Here's how the part is built. I have some questions about the finished solid (model axes, mm). A direction names the side the tool comes from. Round coordinates to 2 decimals unless told otherwise and drop trailing zeros. Order: outer loops, then holes, each group sorted by start corner. A loop starts at its lowest first (then second) coordinate and runs counter-clockwise, first axis right, second up. Notation, with made-up numbers: (34.5, -27) -> (66.5, -27) arc R9 cw to (66.5, -13) -> close; hole circle Ø5 at (-8, -22). An arc over 180 degrees is marked (long way). Answer in a Markdown table with one row per item.
```python
from build123d import *

# Parameters (mm, degrees)
SKETCH1_R           = 22.5
BOSS_EXTRUDE1_DEPTH = 8
CUT_EXTRUDE4_DEPTH  = 111.127199183


with BuildPart() as part:
    # Sketch1 → Boss-Extrude1 (new body)
    with BuildSketch(Plane(origin=(0, 0, 0), x_dir=(1, 0, 0), z_dir=(0, 1, 0))):
        Polygon((10, 0), (35, 0), (35, 8), (60, 8), (60, 92), (35, 92), (35, 100), (10, 100), (10, 92), (0, 92), (0, 8), (10, 8), align=None)
        with Locations(Location((30, 50, 0), (0, 0, 270))):
            Circle(SKETCH1_R, mode=Mode.SUBTRACT)
    extrude(amount=BOSS_EXTRUDE1_DEPTH)

    # Sketch7 → Cut-Extrude4 (cut, through all)
    with BuildSketch(Plane.XY.offset(-8)):
        Polygon((60, 0), (52, 8), (60, 8), align=None)
    extrude(amount=-CUT_EXTRUDE4_DEPTH, mode=Mode.SUBTRACT)


solid = part.part
```
1. Please list where these lines run through material, in increasing order: line 1 along Z through (x, y) = (30, 4.5); line 2 along Z through (x, y) = (28, 5); line 3 along X through (y, z) = (2.5, -50).
Numbers:
| item | result |
|---|---|
| line 1 | z = -100 to -72.5, -27.5 to 0 |
| line 2 | z = -100 to -72.41, -27.59 to 0 |
| line 3 | x = 0 to 7.5, 52.5 to 57.5 |
2. For pin 1 Ø4 at (y, z) = (5.5, -4) entering from -X; pin 2 Ø4 at (x, y) = (5, 6) entering from -Z; pin 3 Ø1.5 at (x, y) = (53, 5) entering from +Z, each with a flat end and sliding along its axis, tell me the tip position at first contact or that it passes through.
Numbers:
| item | result |
|---|---|
| pin 1 | stops at x = 10 |
| pin 2 | stops at z = -92 |
| pin 3 | stops at z = -8 |
3. For faces 1 (the face through (10, 4, -96)), 2 (the face through (10, 4, -4)), 3 (the face through (35, 4, -96)), 4 (the face through (45, 4, -8)), which set-ups out of +Z, -Z, +X, -X, +Y, -Y let a thin tool reach every point of the face, with its end or its side?
Numbers:
| item | result |
|---|---|
| face 1 | -Z, -X, +Y, -Y |
| face 2 | +Z, -X, +Y, -Y |
| face 3 | -Z, +X, +Y, -Y |
| face 4 | +Z, +X, +Y, -Y |
4. Suppose I cut it at B-B on x = 30. Write out the boundary of the cut face in (y, z), then the cut area to 3 significant figures.
Numbers:
| item | result |
|---|---|
| outline | (0, -100) -> (8, -100) -> (8, -72.5) -> (0, -72.5) -> close; (0, -27.5) -> (8, -27.5) -> (8, 0) -> (0, 0) -> close |
| area | 440 mm2 |
5. Suppose I cut it at D-D on y = 6.75. Write out the boundary of the cut face in (x, z), then the cut area to 3 significant figures.
Numbers:
| item | result |
|---|---|
| outline | (0, -92) -> (10, -92) -> (10, -100) -> (35, -100) -> (35, -92) -> (53.25, -92) -> (53.25, -8) -> (35, -8) -> (35, 0) -> (10, 0) -> (10, -8) -> (0, -8) -> close; hole circle Ø45 at (30, -50) |
| area | 3,280 mm2 |
6. Suppose I cut it at C-C on z = -50. Write out the boundary of the cut face in (x, y), then the cut area to 3 significant figures.
Numbers:
| item | result |
|---|---|
| outline | (0, 0) -> (7.5, 0) -> (7.5, 8) -> (0, 8) -> close; (52.5, 0) -> (60, 0) -> (52.5, 7.5) -> close |
| area | 88.1 mm2 |
7. Suppose I cut it at A-A on y = 1. Write out the boundary of the cut face in (x, z), then the cut area to 3 significant figures.
Numbers:
| item | result |
|---|---|
| outline | (0, -92) -> (10, -92) -> (10, -100) -> (35, -100) -> (35, -92) -> (59, -92) -> (59, -8) -> (35, -8) -> (35, 0) -> (10, 0) -> (10, -8) -> (0, -8) -> close; hole circle Ø45 at (30, -50) |
| area | 3,770 mm2 |
